Input: part model. Units: mm. Frame: model coordinates. A direction names the side the tool comes from. Coordinates: 2 decimals unless noted, no trailing zeros. Order: outer loops, then holes, each group sorted by start corner. A loop starts at its lowest first (then second) coordinate and runs counter-clockwise, first axis right, second up. Notation, with made-up numbers: (3, 26) - (54, 26) arc R22 ccw to (54, 63) - close; hole circle Ø5 at (14.25, 48). An arc over 180 degrees is marked (long way). One line per question, with ' | ' between items.
from build123d import *

# Parameters (mm, degrees)
F1_DEPTH = 25.4
F0_W     = 92.877152
F0_H     = 36.552329
F2_DEPTH = 11.1125
F0_W_2   = 13.582083
F0_H_2   = 69.85
F3_DEPTH = 9.525


with BuildPart() as f1:
    # F0 (on Front) → F1 (new body)
    with BuildSketch(Plane.XZ):
        Polygon((27.975522, 5.506429), (-64.90163, 5.506429), (-64.90163, -27.791242), (50.200522, -27.791242), (50.200522, 42.058758), (27.975522, 42.058758), align=None)
    extrude(amount=F1_DEPTH)

    # F0 (on Front) → F2 (join)
    with BuildSketch(Plane.XZ):
        with Locations((-18.463054, 23.782593)):
            Rectangle(F0_W, F0_H)
    extrude(amount=F2_DEPTH)

    # F0 (on Front) → F3 (join)
    with BuildSketch(Plane.XZ):
        with Locations((56.991563, 7.133758)):
            Rectangle(F0_W_2, F0_H_2)
    extrude(amount=F3_DEPTH)


solid = f1.part
Item 1: Access query for faces 1 (the face through (50.201, -17, 7)), 2 (the face through (27.976, -18, 24)), 3 (the face through (5, -25.4, -8)). Directions: +Z, -Z, +X, -X, +Y, -Y. A direction counts if a zero-diameter tool reaches every point of the face in a straight line with its end or side. Return the directions, or none.
Data:
face 1: +Z, -Z, +X, -Y | face 2: +Z, -X, -Y | face 3: +Z, -Z, +X, -X, -Y
Item 2: Section A-A on z = -22. Return the cut outline in (x, y) (3 decimals), and give its area (3 significant figures).
Data:
outline: (-64.902, -25.4) - (50.201, -25.4) - (50.201, -9.525) - (63.783, -9.525) - (63.783, 0) - (-64.902, 0) - close | area: 3,050 mm^2
Item 3: Section B-B on y = -21. Return the cut outline in (x, z), and give its area (4 significant figures).
Data:
outline: (-64.9, -27.79) - (50.2, -27.79) - (50.2, 42.06) - (27.98, 42.06) - (27.98, 5.51) - (-64.9, 5.51) - close | area: 4,645 mm^2
Item 4: Contact query for flat-ended pins moving along their axis: P1, Ø4.5, axis at x = -1.5, y = -20.5, coming from the +Z side; P2, Ø11, axis at x = 57, z = -4, coming from the -Y side (3 decimals); P3, Ø10, axis at x = -47.5, z = 11, coming from the -Y side. Output: stop coordinate, or through.
Data:
P1: z = 5.51 | P2: y = -9.525 | P3: y = -11.11
Item 5: Section C-C on z = 37. Return the cut outline in (x, y) (1 decimal), and give its area (3 significant figures).
Data:
outline: (-64.9, -11.1) - (28, -11.1) - (28, -25.4) - (50.2, -25.4) - (50.2, -9.5) - (63.8, -9.5) - (63.8, 0) - (-64.9, 0) - close | area: 1,730 mm^2
Item 6: Ray query, line 1 (Z direction, x = 5.5, y = -21); line 2 (X direction, y = -15.5, z = 7.5); line 3 (X direction, y = -19.25, z = 4). Return the intervals inside material, ascending.
Data:
line 1: -27.79 to 5.51 | line 2: 27.98 to 50.2 | line 3: -64.9 to 50.2
